Source: CAD feature listing. Evaluate the final solid. Frame: model axes, mm. Coordinates: 2 decimals unless noted, no trailing zeros. Order: outer loops, then holes, each group sorted by start corner. A loop starts at its lowest first (then second) coordinate and runs counter-clockwise, first axis right, second up.
```python
from build123d import *

# Parameters (mm, degrees)
SKETCH_1_W          = 42
SKETCH_1_H          = 26
EXTRUDE_1_DEPTH     = 9.5
SKETCH_3_R          = 4.15
CUT_EXTRUDE_1_DEPTH = 51.301590432
SKETCH_4_R          = 1.9
CUT_EXTRUDE_2_DEPTH = 51.301590432


with BuildPart() as part:
    # 草图1 → 凸台-拉伸1 (new body)
    with BuildSketch(Plane(origin=(0, 0, 0), x_dir=(1, 0, 0), z_dir=(0, 1, 0))):
        with Locations((21, -13)):
            Rectangle(SKETCH_1_W, SKETCH_1_H)
    extrude(amount=EXTRUDE_1_DEPTH)

    # 草图3 → 切除-拉伸1 (cut, through all)
    with BuildSketch(Plane(origin=(0, 9.5, 0), x_dir=(1, 0, 0), z_dir=(0, 1, 0))):
        with Locations(Location((20.47, -8.473805396, 0), (0, 0, 270))):
            Circle(SKETCH_3_R)
    extrude(amount=-CUT_EXTRUDE_1_DEPTH, mode=Mode.SUBTRACT)

    # 草图4 → 切除-拉伸2 (cut, through all)
    with BuildSketch(Plane(origin=(0, 9.5, 0), x_dir=(1, 0, 0), z_dir=(0, 1, 0))):
        with Locations(Location((8, -5, 0), (0, 0, 270))):
            Circle(SKETCH_4_R)
        with Locations(Location((8, -21, 0), (0, 0, 270))):
            Circle(SKETCH_4_R)
        with Locations(Location((34, -5, 0), (0, 0, 270))):
            Circle(SKETCH_4_R)
        with Locations(Location((34, -21, 0), (0, 0, 270))):
            Circle(SKETCH_4_R)
    extrude(amount=-CUT_EXTRUDE_2_DEPTH, mode=Mode.SUBTRACT)


solid = part.part
```
1. Section query A-A on z = 21. Return loops of the section in (x, y), plus the area to 3 significant figures.
Findings:
outline: (0, 0) - (6.1, 0) - (6.1, 9.5) - (0, 9.5) - close; (9.9, 0) - (32.1, 0) - (32.1, 9.5) - (9.9, 9.5) - close; (35.9, 0) - (42, 0) - (42, 9.5) - (35.9, 9.5) - close
area: 327 mm2
2. Section query B-B on x = 8. Return loops of the section in (y, z).
Findings:
outline: (0, 0) - (9.5, 0) - (9.5, 3.1) - (0, 3.1) - close; (0, 6.9) - (9.5, 6.9) - (9.5, 19.1) - (0, 19.1) - close; (0, 22.9) - (9.5, 22.9) - (9.5, 26) - (0, 26) - close
3. Ray query, line 1 (X direction, y = 2.5, z = 21); line 2 (X direction, y = 7, z = 19.5); line 3 (X direction, y = 5.75, z = 8). Return the intervals inside material, ascending.
Findings:
line 1: x = 0 to 6.1, 9.9 to 32.1, 35.9 to 42
line 2: x = 0 to 6.83, 9.17 to 32.83, 35.17 to 42
line 3: x = 0 to 16.35, 24.59 to 42
4. Section query C-C on y = 4.5. Return loops of the section in (x, z).
Findings:
outline: (0, 0) - (42, 0) - (42, 26) - (0, 26) - close; hole circle Ø3.8 at (8, 5); hole circle Ø3.8 at (8, 21); hole circle Ø8.3 at (20.47, 8.47); hole circle Ø3.8 at (34, 5); hole circle Ø3.8 at (34, 21)
5. Draft query along Z for faces 1 (the face through (0, 5, 13)), 2 (the face through (6.844, 4.816, 3.492)), 3 (the face through (32.145, 4.816, 4.588)), 4 (the face through (21, 5, 26)). Return one class per face: released by +Z, released by -Z, zero draft, split by the parting line, or undercut.
Findings:
face 1: zero draft
face 2: undercut
face 3: undercut
face 4: released by +Z
6. Section query D-D on x = 20.47. Return loops of the section in (y, z), plus the area to 3 significant figures.
Findings:
outline: (0, 0) - (9.5, 0) - (9.5, 4.32) - (0, 4.32) - close; (0, 12.62) - (9.5, 12.62) - (9.5, 26) - (0, 26) - close
area: 168 mm2
7. Pin query (flat end, axial travel): P1, Ø3, axis at x = 32, y = 7, coming from the -Z side. Return the tip coordinate at first contact, or that it passes through.
Findings:
P1: stops at z = 0
